from build123d import *

# Parameters (mm, degrees)
EXTRUDE_1_DEPTH      = 46
EXTRUDE_1_DEPTH_BACK = 46
SKETCH_2_R           = 1.6
CUT_EXTRUDE_1_DEPTH  = 5
SKETCH_3_R           = 1.6
CUT_EXTRUDE_2_DEPTH  = 5
SKETCH_4_R           = 1.75
CUT_EXTRUDE_3_DEPTH  = 10
SKETCH_5_R           = 3
CUT_EXTRUDE_4_DEPTH  = 20
SKETCH_6_W           = 108.593038012
SKETCH_6_H           = 21.321920706
CUT_EXTRUDE_5_DEPTH  = 20


with BuildPart() as part:
    # Sketch 1 → Extrude 1 (new body, two sides)
    with BuildSketch(Plane.XY) as extrude_1_sk:
        Polygon((5, 0), (0, 0), (-10.069195574, 12), (-11, 12), (-11, 14), (0, 14), (0, 12), (-7.458380995, 12), (0.932615316, 2), (5, 2), align=None)
    extrude(amount=EXTRUDE_1_DEPTH)
    extrude(extrude_1_sk.sketch, amount=-EXTRUDE_1_DEPTH_BACK)

    # Sketch 2 → Cut-Extrude 1 (cut)
    with BuildSketch(Plane(origin=(0, 14, 0), x_dir=(1, 0, 0), z_dir=(0, 1, 0))):
        with Locations((-2, 41)):
            Circle(SKETCH_2_R)
        with Locations((-2, 35)):
            Circle(SKETCH_2_R)
        with Locations((-2, 3)):
            Circle(SKETCH_2_R)
        with Locations((-2, -3)):
            Circle(SKETCH_2_R)
        with Locations((-2, -35)):
            Circle(SKETCH_2_R)
        with Locations((-2, -41)):
            Circle(SKETCH_2_R)
    extrude(amount=-CUT_EXTRUDE_1_DEPTH, mode=Mode.SUBTRACT)

    # Sketch 3 → Cut-Extrude 2 (cut)
    with BuildSketch(Plane(origin=(0, 2, 0), x_dir=(1, 0, 0), z_dir=(0, 1, 0))):
        with Locations((2.5, 38)):
            Circle(SKETCH_3_R)
        with Locations((2.5, 19)):
            Circle(SKETCH_3_R)
        with Locations((2.5, 0)):
            Circle(SKETCH_3_R)
        with Locations((2.5, -19)):
            Circle(SKETCH_3_R)
        with Locations((2.5, -38)):
            Circle(SKETCH_3_R)
    extrude(amount=-CUT_EXTRUDE_2_DEPTH, mode=Mode.SUBTRACT)

    # Sketch 4 → Cut-Extrude 3 (cut)
    with BuildSketch(Plane(origin=(0, 14, 0), x_dir=(1, 0, 0), z_dir=(0, 1, 0))):
        with Locations((-4.2, 23.75)):
            Circle(SKETCH_4_R)
        with Locations((-4.2, 14.25)):
            Circle(SKETCH_4_R)
        with Locations((-4.2, -14.25)):
            Circle(SKETCH_4_R)
        with Locations((-4.2, -23.75)):
            Circle(SKETCH_4_R)
    extrude(amount=-CUT_EXTRUDE_3_DEPTH, mode=Mode.SUBTRACT)

    # Sketch 5 → Cut-Extrude 4 (cut)
    with BuildSketch(Plane.XZ.offset(-12)):
        with Locations((-4.2, 23.75)):
            Circle(SKETCH_5_R)
        with Locations((-4.2, 14.25)):
            Circle(SKETCH_5_R)
        with Locations((-4.2, -14.25)):
            Circle(SKETCH_5_R)
        with Locations((-4.2, -23.75)):
            Circle(SKETCH_5_R)
    extrude(amount=CUT_EXTRUDE_4_DEPTH, mode=Mode.SUBTRACT)

    # Sketch 6 → Cut-Extrude 5 (cut)
    with BuildSketch(Plane(origin=(0, 0, 0), x_dir=(0, 0, 1), z_dir=(-0.766044443, -0.64278761, 0))):
        with Locations((-2.330535519, 21.720159804)):
            Rectangle(SKETCH_6_W, SKETCH_6_H)
    extrude(amount=CUT_EXTRUDE_5_DEPTH, mode=Mode.SUBTRACT)


solid = part.part
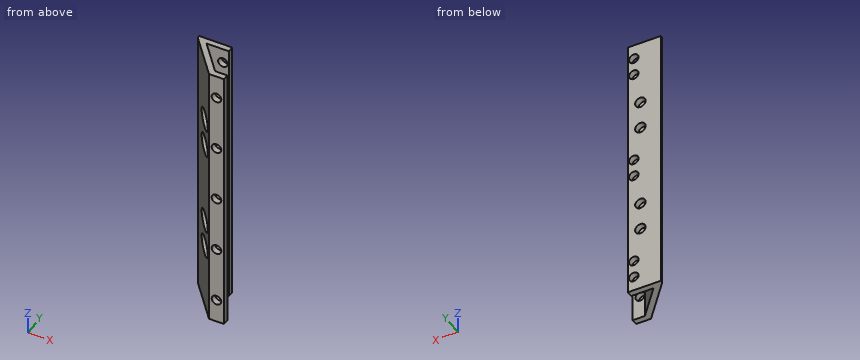
CAD build for the part. Positions are in the model's coordinates, mm. Round coordinates to 2 decimals unless told otherwise and drop trailing zeros. Write each loop counter-clockwise with the first axis right and the second up, starting at its lowest first coordinate (ties: lowest second). Pieces come first, ordered by that corner, then holes.
(1) Drop flat-ended pins along their axis: P1, Ø1, axis at y = 13, z = 20.5, coming from the +X side; P2, Ø5, axis at x = -7, z = 11.5, coming from the -Y side; P3, Ø4, axis at x = -4.2, z = 23.75, coming from the -Y side; P4, Ø2.5, axis at x = 2.5, z = -19, coming from the -Y side. Give the stop position or say it passes through.
(2) Slice it at B-B, the plane z = 35. Write the cut outline in (x, y).
(3) Slice it at A-A, the plane x = 2.5. Write the cut outline in (y, z).
(4) Probe line 1 along Z through (x, y) = (-4.25, 13); line 2 along Z through (x, y) = (2.5, 1.15); line 3 along X through (y, z) = (13.4, 23.75). List the from-to ranges inside material, lowest first.
From the geometry:
1. P1: stops at x = 0
1. P2: stops at y = 5.38
1. P3: stops at y = 12
1. P4: passes through
2. outline: (-11, 13.11) - (0, 0) - (5, 0) - (5, 2) - (0.93, 2) - (-7.46, 12) - (-3.6, 12) - (-3.6, 14) - (-11, 14) - close; (-0.4, 12) - (0, 12) - (0, 14) - (-0.4, 14) - close
3. outline: (0, -46) - (2, -46) - (2, -39.6) - (0, -39.6) - close; (0, -36.4) - (2, -36.4) - (2, -20.6) - (0, -20.6) - close; (0, -17.4) - (2, -17.4) - (2, -1.6) - (0, -1.6) - close; (0, 1.6) - (2, 1.6) - (2, 17.4) - (0, 17.4) - close; (0, 20.6) - (2, 20.6) - (2, 36.4) - (0, 36.4) - close; (0, 39.6) - (2, 39.6) - (2, 46) - (0, 46) - close
4. line 1: z = -46 to -25.5, -22 to -16, -12.5 to 12.5, 16 to 22, 25.5 to 46
4. line 2: z = -46 to -39.6, -36.4 to -20.6, -17.4 to -1.6, 1.6 to 17.4, 20.6 to 36.4, 39.6 to 46
4. line 3: x = -11 to -5.95, -2.45 to 0
